```python
from build123d import *

# Parameters (mm, degrees)
EXTRUDE_1_DEPTH = 10
SKETCH_1_3_R    = 37
SKETCH_1_3_R_2  = 9
SKETCH_1_3_R_3  = 6
EXTRUDE_2_DEPTH = 20


with BuildPart() as part:
    # Sketch 1 → Extrude 1 (new body)
    with BuildSketch(Plane.XY):
        with BuildLine():
            Line((-54.470175326, 37), (-95, 37))
            ThreePointArc((-95, 37), (-68.837049096, 26.162950904), (-58, 0))
            ThreePointArc((-58, 0), (-68.837049096, -26.162950904), (-95, -37))
            Line((-95, -37), (-54.470175326, -37))
            ThreePointArc((-54.470175326, -37), (-48.246282484, -38.260150683), (-43.002769994, -41.842105263))
            ThreePointArc((-43.002769994, -41.842105263), (0, -60), (43.002769994, -41.842105263))
            ThreePointArc((43.002769994, -41.842105263), (48.246282484, -38.260150683), (54.470175326, -37))
            Line((54.470175326, -37), (95, -37))
            ThreePointArc((95, -37), (58, 0), (95, 37))
            Line((95, 37), (54.470175326, 37))
            ThreePointArc((54.470175326, 37), (48.246282484, 38.260150683), (43.002769994, 41.842105263))
            ThreePointArc((43.002769994, 41.842105263), (0, 60), (-43.002769994, 41.842105263))
            ThreePointArc((-43.002769994, 41.842105263), (-48.246282484, 38.260150683), (-54.470175326, 37))
        make_face()
        with BuildLine():
            ThreePointArc((-23.21, 37.380421346), (0, 44), (23.21, 37.380421346))
            ThreePointArc((23.21, 37.380421346), (29.403784815, 28.894964715), (27.951470588, 18.490315372))
            ThreePointArc((27.951470588, 18.490315372), (23, 0), (27.951470588, -18.490315372))
            ThreePointArc((27.951470588, -18.490315372), (29.403784815, -28.894964715), (23.21, -37.380421346))
            ThreePointArc((23.21, -37.380421346), (0, -44), (-23.21, -37.380421346))
            ThreePointArc((-23.21, -37.380421346), (-29.403784815, -28.894964715), (-27.951470588, -18.490315372))
            ThreePointArc((-27.951470588, -18.490315372), (-23, 0), (-27.951470588, 18.490315372))
            ThreePointArc((-27.951470588, 18.490315372), (-29.403784815, 28.894964715), (-23.21, 37.380421346))
        make_face(mode=Mode.SUBTRACT)
    extrude(amount=EXTRUDE_1_DEPTH)

    # Sketch 1_3 → Extrude 2 (add)
    # profile 1 of 2: a face of its own
    with BuildSketch(Plane.XY):
        with Locations(Location((95, 0, 0), (0, 0, 270))):
            Circle(SKETCH_1_3_R)
        with Locations((95, 0)):
            Circle(SKETCH_1_3_R_2, mode=Mode.SUBTRACT)
        with Locations((95, 24)):
            Circle(SKETCH_1_3_R_3, mode=Mode.SUBTRACT)
        with Locations((115.784609691, -12)):
            Circle(SKETCH_1_3_R_3, mode=Mode.SUBTRACT)
        with Locations((74.215390309, -12)):
            Circle(SKETCH_1_3_R_3, mode=Mode.SUBTRACT)
    # profile 2 of 2: a face of its own
    with BuildSketch(Plane.XY):
        with Locations(Location((-95, 0, 0), (0, 0, 90))):
            Circle(SKETCH_1_3_R)
        with Locations((-95, 0)):
            Circle(SKETCH_1_3_R_2, mode=Mode.SUBTRACT)
        with Locations((-95, 23)):
            Circle(SKETCH_1_3_R_3, mode=Mode.SUBTRACT)
        with Locations((-73.125700125, 7.107390871)):
            Circle(SKETCH_1_3_R_3, mode=Mode.SUBTRACT)
        with Locations((-81.480939197, -18.607390871)):
            Circle(SKETCH_1_3_R_3, mode=Mode.SUBTRACT)
        with Locations((-108.519060803, -18.607390871)):
            Circle(SKETCH_1_3_R_3, mode=Mode.SUBTRACT)
        with Locations((-116.874299875, 7.107390871)):
            Circle(SKETCH_1_3_R_3, mode=Mode.SUBTRACT)
    extrude(amount=EXTRUDE_2_DEPTH)


solid = part.part
```
Geometry: final body of the model. Coordinates: model frame, mm. A direction names the side the tool comes from. Coordinates: 2 decimals unless noted, no trailing zeros. Write each loop counter-clockwise with the first axis right and the second up, starting at its lowest first coordinate (ties: lowest second). Pieces come first, ordered by that corner, then holes. Notation, with made-up numbers: M 14.5,-19.5 L 24.5,-19.5 A16 cw 24.5,4.5 Z; hole C 59.25,53 d8. An arc over 180 degrees is marked long. Answer as CSV lines item,"result". Start each with the question number.
Q1. Cut plane C-C on y = -22. Return the cut outline in (x, z).
Q2. Cut plane B-B on z = 17.25. Count the separate pieces of the cut face and the enclosed holes in it, then the cut area to 3 significant figures.
Q3. Line query: line 1 (Y direction, x = -95, z = 9.5); line 2 (X direction, y = -19.5, z = 12); line 3 (Z direction, x = -51.5, y = 8). Output: solid intervals per line, ascending. Write a range as from..to.
Q4. Pin query (flat end, axial travel): P1, Ø8, axis at x = -73.5, z = 7.5, coming from the -Y side; P2, Ø6, axis at y = -3.5, z = 7, coming from the -X side; P3, Ø12, axis at x = -81, z = 15, coming from the +Y side. Return the tip coordinate at first contact, or that it passes through.
Q5. Reachability of faces 4 (the cylindrical face through (-29.366, -29.041, 4.93)), 5 (the flat face through (74, -37, 5)), 6 (the cylindrical face through (-131.685, -4.817, 12.082)), 7 (the cylindrical face through (48.329, 38.226, 4.93)), 8 (the flat face through (-75, -37, 5)) from +Z, -Z, +X, -X, +Y, -Y: full face, straight path, thin tool, end or side. Return the list, or none.
Q6. Cut plane A-A on x = -7. Return the cut outline in (y, z).
Q7. Mould query, pull axis X, two halves, no side actions, for faces 1 (the flat face through (-29, -4, 10)), 2 (the cylindrical face through (48.164, -38.295, 4.93)), 3 (the flat face through (87, -8, 20)). Classes: released by +X, released by -X, zero draft, split by the parting line, or undercut.
Findings below:
1,outline,"M -124.75,0 L -113.47,0 L -113.47,20 L -124.75,20 Z; M -103.57,0 L -86.43,0 L -86.43,20 L -103.57,20 Z; M -76.53,0 L -29.38,0 L -29.38,10 L -65.25,10 L -65.25,20 L -76.53,20 Z; M 29.38,0 L 124.75,0 L 124.75,20 L 65.25,20 L 65.25,10 L 29.38,10 Z"
2,separate pieces,"2"
2,enclosed holes,"10"
2,area,"7,190 mm2"
3,line 1,"y = -37..-9, 9..17, 29..37"
3,line 2,"x = -126.44..-114.45, -102.59..-87.41, -75.55..-63.56, 63.56..126.44"
3,line 3,"z = 0..10"
4,P1,"stops at y = -37"
4,P2,"stops at x = -132"
4,P3,"stops at y = 37"
5,face 4,"+Z, -Z"
5,face 5,"+Z, -Z, +X, -Y"
5,face 6,"+Z"
5,face 7,"+Z, -Z, +X, +Y"
5,face 8,"+Z, -Z, -X, -Y"
6,outline,"M -59.59,0 L -43.44,0 L -43.44,10 L -59.59,10 Z; M 43.44,0 L 59.59,0 L 59.59,10 L 43.44,10 Z"
7,face 1,"undercut"
7,face 2,"released by +X"
7,face 3,"zero draft"
